Job drawing, mm, ordinate dimensions from the low corner. One solid piece. A direction names the side the tool comes from. Coordinates: 2 decimals unless noted, no trailing zeros. Loops run counter-clockwise (first coordinate to the right, second up) from the corner with the lowest first, then second, coordinate; pieces in that order, holes last. Notation, with made-up numbers: (68, 37.5) - (116, 37.5) arc R14 ccw to (116, 51.5) - close; hole circle Ø7 at (-21, 7). An arc over 180 degrees is marked (long way). Use a Markdown table: item, result. Add a question column.
1) Tool access for the marked faces 1, 2, 3 and 4: list every direction of +Z, -Z, +X, -X, +Y, -Y with a clear straight run to the whole face (end or side of a thin tool).
2) Band-saw the part on C-C (x = 5). Give the cut face in (y, z) (1 decimal), plus the area to 3 significant figures.
3) Probe probe 1 along X at (y, z) = (6, 19) (1 decimal); probe 2 along Z at (x, y) = (24.5, 4) (1 decimal); probe 3 along X at (y, z) = (4.75, 14) (1 decimal). List the from-to ranges inside material, lowest first. Write a range as [from, to].
4) Drop flat-ended pins along their axis: P1, Ø6, axis at x = 8.5, z = 27.5, coming from the -Y side; P2, Ø1.1, axis at x = 24.6, z = 19.1, coming from the -Y side; P3, Ø2.5, axis at x = 22, z = 30, coming from the -Y side (3 decimals); P4, Ø6, axis at x = 3.5, z = 19, coming from the +Y side (3 decimals). Give the stop position or say it passes through.
5) Band-saw the part on A-A (y = 2.25). Give the cut face in (x, z) (1 decimal), plus the area to 3 significant figures.
6) Pull direction Z, two halves, no side cores. Call the marked faces 5, 6 and 7: +Z half, -Z half, draft (parallel to the pull), parting line (faces both ways), or undercut.
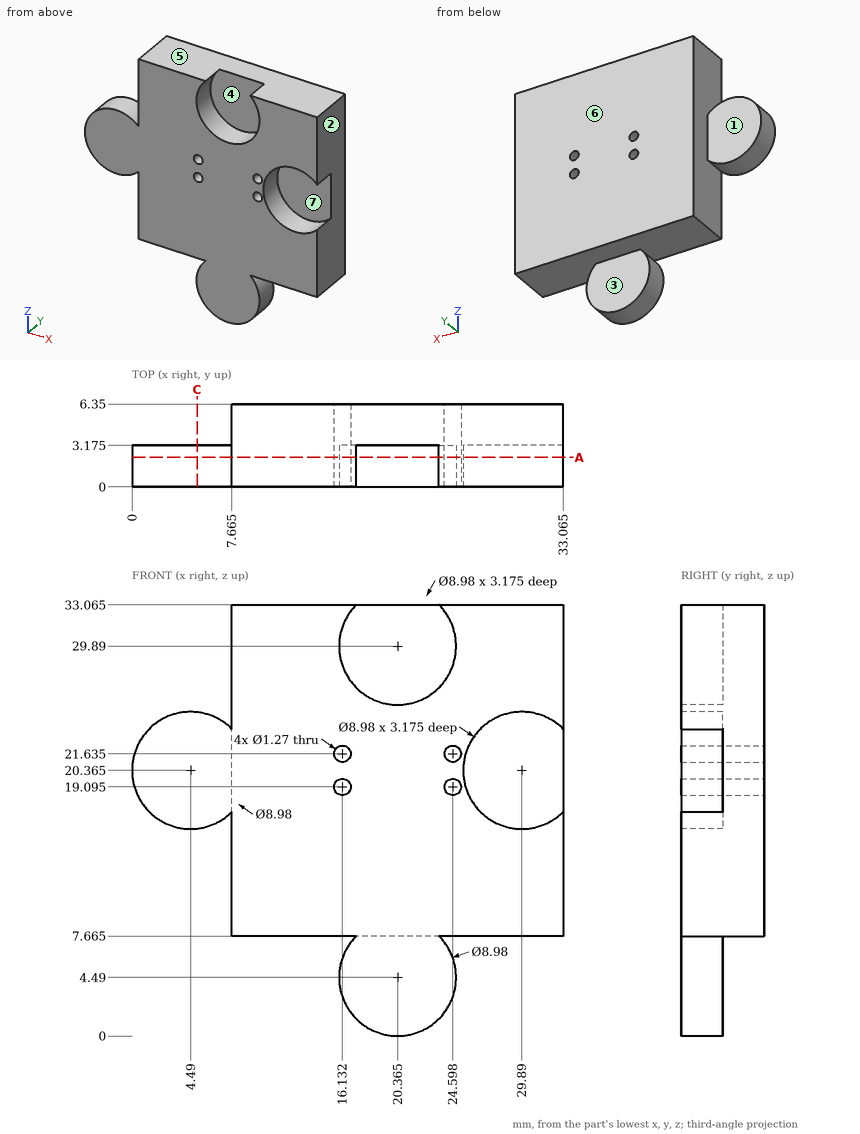
Answer block:
| question | item | result |
|---|---|---|
| 1 | face 1 | +Z, -Z, -X, +Y |
| 1 | face 2 | +Z, -Z, +X, +Y, -Y |
| 1 | face 3 | -Z, +X, -X, +Y |
| 1 | face 4 | -Y |
| 2 | outline | (0, 15.9) - (3.2, 15.9) - (3.2, 24.8) - (0, 24.8) - close |
| 2 | area | 28.3 mm2 |
| 3 | probe 1 | [7.7, 15.5], [16.8, 24], [25.2, 33.1] |
| 3 | probe 2 | [7.7, 18.5], [19.7, 21], [22.3, 33.1] |
| 3 | probe 3 | [7.7, 33.1] |
| 4 | P1 | y = 0 |
| 4 | P2 | through |
| 4 | P3 | y = 3.175 |
| 4 | P4 | y = 3.175 |
| 5 | outline | (7.7, 7.7) - (17.2, 7.7) arc R4.5 ccw (long way) to (23.5, 7.7) - (33.1, 7.7) - (33.1, 17.2) arc R4.5 cw (long way) to (33.1, 23.5) - (33.1, 33.1) - (23.5, 33.1) arc R4.5 cw (long way) to (17.2, 33.1) - (7.7, 33.1) - (7.7, 23.5) arc R4.5 ccw (long way) to (7.7, 17.2) - close; hole circle Ø1.3 at (16.1, 19.1); hole circle Ø1.3 at (16.1, 21.6); hole circle Ø1.3 at (24.6, 19.1); hole circle Ø1.3 at (24.6, 21.6) |
| 5 | area | 640 mm2 |
| 6 | face 5 | +Z half |
| 6 | face 6 | draft |
| 6 | face 7 | undercut |
